Input: dimensioned drawing with shaded views. Units: mm. Origin: part minimum x, y, z. Give positions to 0.01 mm unless a question says otherwise; leave off trailing zeros. Write each loop counter-clockwise with the first axis right and the second up, starting at its lowest first coordinate (ties: lowest second). Pieces come first, ordered by that corner, then holes. Notation, with made-up numbers: (-34, -21.5) -> (14, -21.5) arc R7 cw to (14, -10.5) -> close; hole circle Ø11 at (65.5, -23). An arc over 180 degrees is marked (long way). Answer as a JSON object with one key per item and string values. Group by question number.
(1) Section query D-D on y = 27. Output: boundary loops of the cut face in (x, z), plus the area to 3 significant figures.
(2) Material intervals for probe 1 along Y at (x, z) = (30.5, 33.5); probe 2 along Y at (x, z) = (9.5, 8); probe 3 along Z at (x, y) = (42, 17), sorted ascending.
(3) Contact query for flat-ended pins moving along their axis: pin 1 Ø8 at (x, y) = (40, 33.5) entering from +Z; pin 2 Ø4 at (x, z) = (61.5, 34.5) entering from +Y; pin 3 Ø1 at (y, z) = (12, 36.5) entering from +X. Output: stop coordinate, or through.
(4) Section query A-A on z = 7. Output: boundary loops of the cut face in (x, y), plus the area to 4 significant figures.
(5) Section query C-C on x = 68. Output: boundary loops of the cut face in (y, z).
(6) Section query B-B on y = 20. Output: boundary loops of the cut face in (x, z), plus the area to 3 significant figures.
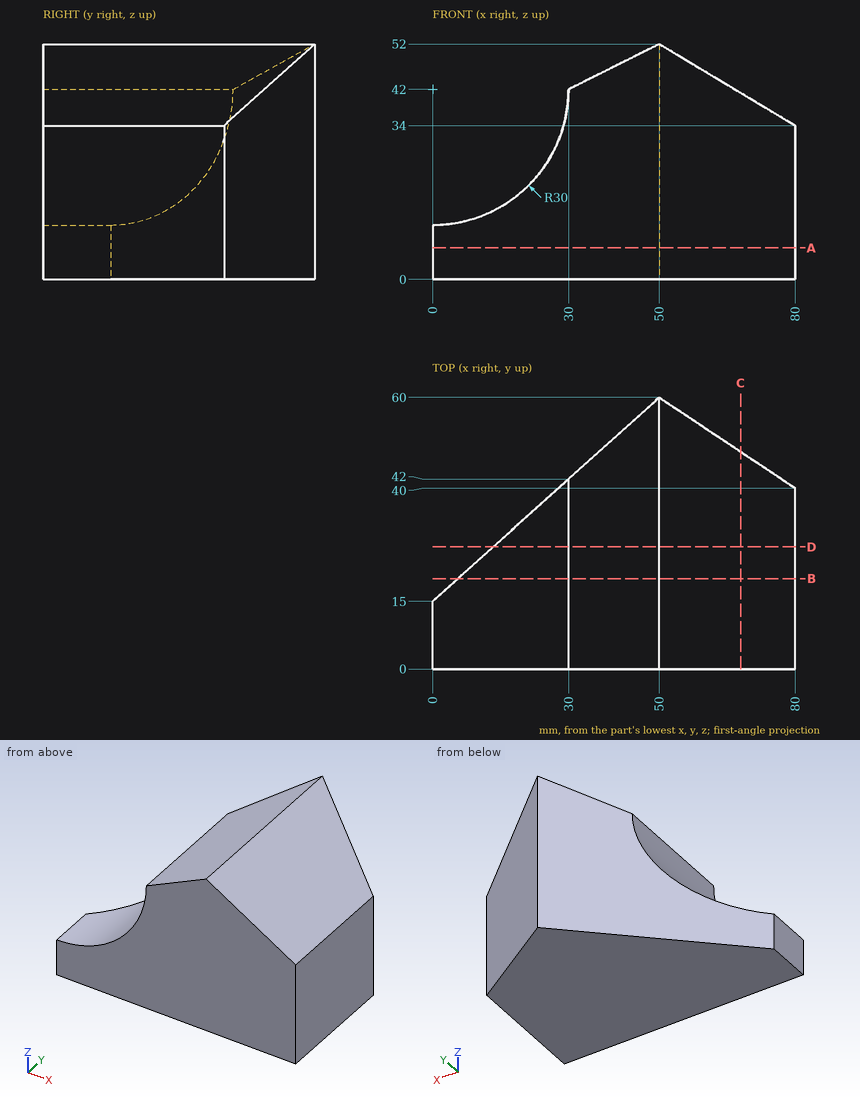
Answer list:
{
 "1": {"outline": "(13.33, 0) -> (80, 0) -> (80, 34) -> (50, 52) -> (30, 42) arc R30 cw to (13.33, 15.13) -> close", "area": "2,610 mm2"},
 "2": {"probe 1": "0 to 42.45", "probe 2": "0 to 23.55", "probe 3": "0 to 48"},
 "3": {"pin 1": "z = 49", "pin 2": "y = 53.67", "pin 3": "x = 76.67"},
 "4": {"outline": "(0, 0) -> (80, 0) -> (80, 40) -> (50, 60) -> (0, 15) -> close", "area": "3,375 mm2"},
 "5": {"outline": "(0, 0) -> (48, 0) -> (48, 41.2) -> (0, 41.2) -> close"},
 "6": {"outline": "(5.56, 0) -> (80, 0) -> (80, 34) -> (50, 52) -> (30, 42) arc R30 cw to (5.56, 12.52) -> close", "area": "2,720 mm2"}
}
